Autodesk Inventor part; units mm, degrees
ref_plane "YZ Plane" through (0, 0, 0) normal (1, 0, 0) x (0, 1, 0)
ref_plane "XZ Plane" through (0, 0, 0) normal (0, 1, 0) x (-1, 0, 0)
ref_plane "XY Plane" through (0, 0, 0) normal (0, 0, 1) x (1, 0, 0)
sketch "Sketch1" plane through (0, 0, 0) normal (0, 0, 1) x (1, 0, 0)
  line L0 (-6.6884, 12.6835) -> (43.3116, 12.6835)
  line L1 (43.3116, 12.6835) -> (43.3116, -37.3165)
  line L2 (43.3116, -37.3165) -> (-6.6884, -37.3165)
  line L3 (-6.6884, -37.3165) -> (-6.6884, 12.6835)
  point P0 (0, 0)
  dimension "d0" = 50
  dimension "d1" = 50
extrude "Extrusion1" add sketch "Sketch1" along normal blind 41
sketch "Sketch2" plane through (0, 0, 41) normal (0, 0, 1) x (1, 0, 0)
  circle A0 centre (18.3116, -12.3165) radius 21
  point P0 (0, 0)
  dimension "d4" = 42
extrude "Extrusion2" add sketch "Sketch2" along normal blind 29
sketch "Sketch3" plane through (18.3116, -12.3165, 70) normal (0, 0, 1) x (1, 0, 0)
  circle A0 centre (0, 0) radius 21
  circle A1 centre (0, 0) radius 6.35
  point P0 (-18.3116, 12.3165)
  dimension "d7" = 12.7
extrude "Extrusion3" cut sketch "Sketch3" against normal blind 29 contours A1
sketch "Sketch4" plane through (18.3116, -12.3165, 41) normal (0, 0, 1) x (1, 0, 0)
  circle A0 centre (0, 0) radius 6.35
  point P0 (-18.3116, 12.3165)
extrude "Extrusion4" add sketch "Sketch4" along normal blind 21
sketch "Sketch5" plane through (18.3116, -12.3165, 62) normal (0, 0, 1) x (1, 0, 0)
  circle A0 centre (0, 0) radius 6.35
  point P0 (-18.3116, 12.3165)
extrude "Extrusion5" cut sketch "Sketch5" against normal blind 1
sketch "Sketch6" plane through (18.3116, -12.3165, 61) normal (0, 0, 1) x (1, 0, 0)
  circle A0 centre (0, 0) radius 6.35
  line L0 (-6.35, 0) -> (6.35, 0)
  point P0 (-18.3116, 12.3165)
extrude "Extrusion6" add sketch "Sketch6" along normal blind 8 contours L0 A0 picked at (1.8268, 2.3873)
sketch "Sketch7" plane through (18.3116, -12.3165, 69) normal (0, 0, 1) x (1, 0, 0)
  arc A0 (6.35, 0) -> (-6.35, 0) centre (0, 0) ccw
  line L0 (6.35, 0) -> (-6.35, 0)
  point P0 (-18.3116, 12.3165)
extrude "Extrusion7" add sketch "Sketch7" along normal blind 1
sketch "Sketch8" plane through (0, 0, 0) normal (0, 0, -1) x (-1, 0, 0)
  line L0 (-43.3116, 12.6835) -> (-38.3116, 12.6835)
  line L1 (-38.3116, 12.6835) -> (-38.3116, 7.6835)
  line L2 (-38.3116, 7.6835) -> (-43.3116, 7.6835)
  line L3 (-43.3116, 7.6835) -> (-43.3116, 12.6835)
  line L4 (6.6884, -37.3165) -> (1.6884, -37.3165)
  line L5 (1.6884, -37.3165) -> (1.6884, -32.3165)
  line L6 (1.6884, -32.3165) -> (6.6884, -32.3165)
  line L7 (6.6884, -32.3165) -> (6.6884, -37.3165)
  line L8 (-38.3116, 7.6835) -> (1.6884, 7.6835)
  line L9 (1.6884, 7.6835) -> (1.6884, -32.3165)
  line L10 (1.6884, -32.3165) -> (-38.3116, -32.3165)
  line L11 (-38.3116, -32.3165) -> (-38.3116, 7.6835)
  circle A0 centre (-38.3116, -32.3165) radius 0.5
  circle A1 centre (1.6884, 7.6835) radius 0.5
  point P0 (0, 0)
  dimension "d18" = 5
  dimension "d19" = 5
  dimension "d20" = 5
  dimension "d21" = 5
  dimension "d22" = 1
  dimension "d23" = 1
extrude "Extrusion8" cut sketch "Sketch8" against normal blind 6 contours A1 L9 L8 | L8 L9 A1 | A0 L10 L11 | L11 L10 A0
properties part number "hmodel"
Input: part model. Units: mm. Frame: model coordinates. A direction names the side the tool comes from. Coordinates: 2 decimals unless noted, no trailing zeros. Write each loop counter-clockwise with the first axis right and the second up, starting at its lowest first coordinate (ties: lowest second). Pieces come first, ordered by that corner, then holes. Notation, with made-up numbers: (80.5, -29) -> (99.5, -29) arc R16 ccw to (99.5, -7) -> close; hole circle Ø10 at (-31.5, 43). An arc over 180 degrees is marked (long way). Answer as a JSON object with one key per item and string values.
1. Access query for faces 4 (the face through (40, -12, 41)), 5 (the face through (-6.688, -13, 20)). Directions: +Z, -Z, +X, -X, +Y, -Y. A direction counts if a zero-diameter tool reaches every point of the face in a straight line with its end or side. Return the directions, or none.
Result set:
{"face 4": "+Z", "face 5": "+Z, -Z, -X, +Y, -Y"}
2. First-contact query: P1, Ø1.5, axis at x = 24, y = 6, coming from the -Z side; P2, Ø3, axis at x = -0.5, y = -26, coming from the +Z side; P3, Ø1.5, axis at x = 31.5, z = 59.5, coming from the +Y side; P4, Ø10, axis at x = 21.5, z = 48, coming from the -Y side. Flat tips, straight axial feed; report the tip coordinate or a pass-through.
Result set:
{"P1": "stops at z = 0", "P2": "stops at z = 41", "P3": "stops at y = 4.6", "P4": "stops at y = -33.32"}
3. Section A-A on y = 2.5. Return the cut outline in (x, z), then the cut area to 3 significant figures.
Result set:
{"outline": "(-6.69, 0) -> (43.31, 0) -> (43.31, 41) -> (33.19, 41) -> (33.19, 70) -> (3.43, 70) -> (3.43, 41) -> (-6.69, 41) -> close", "area": "2,910 mm2"}
4. Section D-D on z = 55.5. Return the cut outline in (x, y), then the cut area to 3 significant figures.
Result set:
{"outline": "circle Ø42 at (18.31, -12.32)", "area": "1,390 mm2"}
5. Mould query, pull axis Y, two halves, no side actions, for faces 1 (the face through (19, -37.316, 20)), 2 (the face through (18, -12, 70)), 3 (the face through (18.172, -18.665, 65.563)). Classes: released by +Y, released by -Y, zero draft, split by the parting line, or undercut.
Result set:
{"face 1": "released by -Y", "face 2": "zero draft", "face 3": "undercut"}
6. Section B-B on x = 33.5. Return the cut outline in (y, z), then the cut area to 3 significant figures.
Result set:
{"outline": "(-37.32, 0) -> (12.68, 0) -> (12.68, 41) -> (2.19, 41) -> (2.19, 70) -> (-26.82, 70) -> (-26.82, 41) -> (-37.32, 41) -> close", "area": "2,890 mm2"}
7. Material intervals for line 1 (Z direction, x = 17.5, y = -18.5); line 2 (Z direction, x = 3, y = 3); line 3 (X direction, y = -4.5, z = 50), sorted ascending. Write a range as from..to.
Result set:
{"line 1": "z = 0..61", "line 2": "z = 0..41", "line 3": "x = -1.18..37.8"}
8. Section C-C on z = 63.5. Return the cut outline in (x, y).
Result set:
{"outline": "circle Ø42 at (18.31, -12.32); hole (11.96, -12.32) arc R6.35 ccw to (24.66, -12.32) -> close"}
